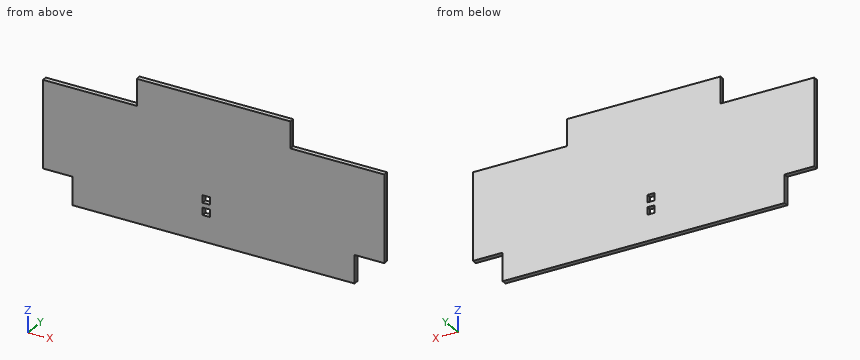
from build123d import *

# Parameters (mm, degrees)
EXTRUDE_1_DEPTH     = 1.6
SKETCH_2_W          = 2.4
SKETCH_2_H          = 2.5
CUT_EXTRUDE_1_DEPTH = 10


with BuildPart() as part:
    # 草图1 → 凸台-拉伸1 (new body)
    with BuildSketch(Plane(origin=(0, 0, 0), x_dir=(1, 0, 0), z_dir=(0, 1, 0))):
        Polygon((-115, 9), (-83.4, 9), (-83.4, 0), (-31.6, 0), (-31.6, 9), (0, 9), (0, 38.5), (-10, 38.5), (-10, 48), (-105, 48), (-105, 38.5), (-115, 38.5), align=None)
    extrude(amount=EXTRUDE_1_DEPTH)

    # 草图2 → 切除-拉伸1 (cut)
    with BuildSketch(Plane(origin=(0, 1.6, 0), x_dir=(1, 0, 0), z_dir=(0, 1, 0))):
        with Locations((-60, 38)):
            Rectangle(SKETCH_2_W, SKETCH_2_H)
        with Locations((-60, 33.9)):
            Rectangle(SKETCH_2_W, SKETCH_2_H)
    extrude(amount=-CUT_EXTRUDE_1_DEPTH, mode=Mode.SUBTRACT)


solid = part.part
For this review, take the finished solid that the model builds, in its own axes (mm). Give positions to 0.01 mm unless a question says otherwise; leave off trailing zeros. Loops run counter-clockwise (first coordinate to the right, second up) from the corner with the lowest first, then second, coordinate; pieces in that order, holes last. Notation, with made-up numbers: M 10,1 L 23,1 A12 ccw 23,18 Z; hole C 28,-37 d3. An arc over 180 degrees is marked long. Answer as a JSON object with one key per item and string values. Group by question number.
Q1. For probe 1 along X at (y, z) = (1.35, -37); probe 2 along X at (y, z) = (0.45, -40); probe 3 along Z at (x, y) = (-16, 0.1), list the stretches that pass through material, from the lowest coordinate up. Write a range as [from, to].
Q2. Add section A-A on y = 0.7. Give the boundary of the cut face in (x, z), and give its area (3 significant figures).
Q3. Add section B-B on z = -4.5. Give the boundary of the cut face in (x, y).
Q4. Add section C-C on x = -15. Give the boundary of the cut face in (y, z).
Q5. Insertion check: P1, Ø0.8, axis at x = -17.5, y = 1, coming from the +Z side; P2, Ø1.5, axis at x = -14.5, z = -8, coming from the +Y side; P3, Ø0.5, axis at y = 1, z = -45, coming from the -X side; P4, Ø0.5, axis at x = -60, y = 0.5, coming from the +Z side. Each pin has a flat end and moves straight along its axis. Give the tip position at first contact, or say it passes through.
Checked values:
{
 "1": {"probe 1": "[-115, -61.2], [-58.8, 0]", "probe 2": "[-105, -10]", "probe 3": "[-48, -9]"},
 "2": {"outline": "M -115,-38.5 L -105,-38.5 L -105,-48 L -10,-48 L -10,-38.5 L 0,-38.5 L 0,-9 L -31.6,-9 L -31.6,0 L -83.4,0 L -83.4,-9 L -115,-9 Z; hole M -61.2,-39.25 L -58.8,-39.25 L -58.8,-36.75 L -61.2,-36.75 Z; hole M -61.2,-35.15 L -58.8,-35.15 L -58.8,-32.65 L -61.2,-32.65 Z", "area": "4,750 mm²"},
 "3": {"outline": "M -83.4,0 L -31.6,0 L -31.6,1.6 L -83.4,1.6 Z"},
 "4": {"outline": "M 0,-48 L 1.6,-48 L 1.6,-9 L 0,-9 Z"},
 "5": {"P1": "z = -9", "P2": "through", "P3": "x = -105", "P4": "z = 0"}
}
